from build123d import *

# Parameters (mm, degrees)
BOSS_EXTRUDE1_DEPTH      = 5
BOSS_EXTRUDE1_DEPTH_BACK = 2
SKETCH3_W                = 30
SKETCH3_H                = 10
BOSS_EXTRUDE2_DEPTH      = 25
SKETCH4_R                = 2.5
CUT_EXTRUDE1_DEPTH       = 83.331203834
RIB1_REACH               = 76.683
SKETCH6_WALL_W           = 186.72160491
SKETCH6_WALL_H           = 5
CUT_EXTRUDE2_DEPTH       = 7
CUT_EXTRUDE3_DEPTH       = 5
FILLET1_R                = 4
SKETCH9_R                = 1.75
CUT_EXTRUDE4_DEPTH       = 60.485369609
CHAMFER1_SIZE            = 1.6
FILLET2_R                = 4
SKETCH10_R               = 1.6
CUT_EXTRUDE5_DEPTH       = 52.293180378
CUT_EXTRUDE6_DEPTH       = 4
CHAMFER2_SIZE            = 1.6
FILLET3_R                = 2


with BuildPart() as part:
    # Sketch1 → Boss-Extrude1 (new, two sides)
    with BuildSketch(Plane.XY) as boss_extrude1_sk:
        Polygon((15, 27.5), (15, 12.5), (43.284271247, -15.784271247), (23.284271247, -35.784271247), (15, -27.5), (-15, -27.5), (-15, 27.5), align=None)
    extrude(amount=BOSS_EXTRUDE1_DEPTH)
    extrude(boss_extrude1_sk.sketch, amount=-BOSS_EXTRUDE1_DEPTH_BACK)

    # Sketch3 → Boss-Extrude2 (add)
    with BuildSketch(Plane.XY.offset(5)):
        with Locations((0, 22.5)):
            Rectangle(SKETCH3_W, SKETCH3_H)
    extrude(amount=BOSS_EXTRUDE2_DEPTH)

    # Sketch4 → Cut-Extrude1 (cut, through all)
    with BuildSketch(Plane(origin=(0, 27.5, 0), x_dir=(1, 0, 0), z_dir=(0, 1, 0))):
        with Locations(Location((-5, -13.9175, 0), (0, 0, 270))):
            Circle(SKETCH4_R)
    extrude(amount=-CUT_EXTRUDE1_DEPTH, mode=Mode.SUBTRACT)

    # Sketch6 wall → Rib1 (add, up to next)
    with BuildSketch(Plane(origin=(-15, 5, 17.5), x_dir=(0, -0.707106781187, -0.707106781187), z_dir=(0, -0.707106781187, 0.707106781187)), mode=Mode.PRIVATE) as rib1_sk1:
        with Locations((0, 2.5)):
            Rectangle(SKETCH6_WALL_W, SKETCH6_WALL_H)
    rib1_tool1 = extrude(rib1_sk1.sketch, amount=-RIB1_REACH, mode=Mode.PRIVATE) - part.part
    add(rib1_tool1.solids().sort_by_distance((-15, 5, 17.5))[0])

    # Sketch7 → Cut-Extrude2 (cut)
    with BuildSketch(Plane.XY.offset(5)):
        with BuildLine():
            Line((22.174744155, -18.158867896), (26.819805153, -32.248737342))
            Line((26.819805153, -32.248737342), (23.284271247, -35.784271247))
            Line((23.284271247, -35.784271247), (-15, -27.5))
            Line((-15, -27.5), (-15, -7.855339059))
            Line((-15, -7.855339059), (7.928932188, -7.855339059))
            ThreePointArc((7.928932188, -7.855339059), (16.719635588, -10.701182004), (22.174744155, -18.158867896))
        make_face()
    extrude(amount=-CUT_EXTRUDE2_DEPTH, mode=Mode.SUBTRACT)

    # Sketch8 → Cut-Extrude3 (cut)
    with BuildSketch(Plane(origin=(0, 17.5, 0), x_dir=(-1, 0, 0), z_dir=(0, -1, 0))):
        Polygon((0.265727793, -13.9175), (2.632863896, -18.0175), (7.367136104, -18.0175), (9.734272207, -13.9175), (7.367136104, -9.8175), (2.632863896, -9.8175), align=None)
    extrude(amount=-CUT_EXTRUDE3_DEPTH, mode=Mode.SUBTRACT)

    # Fillet1
    fillet1_edges = [part.edges().sort_by_distance(p)[0] for p in [
        (-15, 22.5, 30),
        (15, 22.5, 30),
    ]]
    fillet(fillet1_edges, radius=FILLET1_R)

    # Sketch9 → Cut-Extrude4 (cut, through all)
    with BuildSketch(Plane.XY.offset(5)):
        with Locations((15, -1.642135624)):
            Circle(SKETCH9_R)
        with Locations((29.142135624, -15.784271247)):
            Circle(SKETCH9_R)
        with Locations((-2.071067812, 2.5)):
            Circle(SKETCH9_R)
    extrude(amount=-CUT_EXTRUDE4_DEPTH, mode=Mode.SUBTRACT)

    # Chamfer1
    chamfer1_edges = [part.edges().sort_by_distance(p)[0] for p in [
        (-3.821067812, 2.5, 5),
        (27.392135624, -15.784271247, 5),
        (13.25, -1.642135624, 5),
    ]]
    chamfer(chamfer1_edges, length=CHAMFER1_SIZE)

    # Fillet2
    fillet2_edges = [part.edges().sort_by_distance(p)[0] for p in [
        (15, 12.5, 1.5),
        (43.284271247, -15.784271247, 1.5),
        (26.819805153, -32.248737342, 1.5),
        (-15, -7.855339059, 1.5),
    ]]
    fillet(fillet2_edges, radius=FILLET2_R)

    # Sketch10 → Cut-Extrude5 (cut, through all)
    with BuildSketch(Plane(origin=(15, 0, 0), x_dir=(0, 0, -1), z_dir=(1, 0, 0))):
        with Locations(Location((-7, 22.5, 0), (0, 0, 90))):
            Circle(SKETCH10_R)
    extrude(amount=-CUT_EXTRUDE5_DEPTH, mode=Mode.SUBTRACT)

    # Sketch11 → Cut-Extrude6 (cut)
    with BuildSketch(Plane.ZY.offset(15)):
        Polygon((8.58771324, 19.75), (10.175426481, 22.5), (8.58771324, 25.25), (5.41228676, 25.25), (3.824573519, 22.5), (5.41228676, 19.75), align=None)
    extrude(amount=-CUT_EXTRUDE6_DEPTH, mode=Mode.SUBTRACT)

    # Chamfer2
    chamfer2_edges = [part.edges().sort_by_distance(p)[0] for p in [
        (15, 20.9, 7),
    ]]
    chamfer(chamfer2_edges, length=CHAMFER2_SIZE)

    # Fillet3
    fillet3_edges = [part.edges().sort_by_distance(p)[0] for p in [
        (-10, 5, 5),
    ]]
    fillet(fillet3_edges, radius=FILLET3_R)


solid = part.part
Geometry check sheet. Reference: the model listing, model coordinates, mm. A direction names the side the tool comes from. Round coordinates to 2 decimals unless told otherwise and drop trailing zeros. Loops run counter-clockwise (first coordinate to the right, second up) from the corner with the lowest first, then second, coordinate; pieces in that order, holes last. Notation, with made-up numbers: (66.5, 46) - (111.5, 46) arc R20 ccw to (111.5, 74) - close; hole circle Ø5 at (54.5, 19). An arc over 180 degrees is marked (long way). One line per question, with ' | ' between items. Start each with the question number.
1. Depth check by flat-ended pin: pin 1 (12 mm diameter, centred on x = -3.5, z = 8.5, fed in from -Y); pin 2 (14 mm diameter, centred on x = 19.5, y = 3, fed in from +Z); pin 3 (10 mm diameter, centred on x = 3.5, z = 21, fed in from -Y); pin 4 (4 mm diameter, centred on x = -5, z = 13.92, fed in from +Y). Enter the tip coordinate at first touch or a pass-through.
2. Cross-section at D-D on z = 0.5. Record the cut outline in (x, y).
3. Cross-section at C-C on z = 23. Record the cut outline in (x, y), then the cut area to 3 significant figures.
4. Draft check along Z on faces 4 (the face through (-7, 22.5, 12)), 5 (the face through (0, 27.5, 14)), 6 (the face through (0, 23, 30)). Enter one of: released by +Z, released by -Z, zero draft, split by the parting line, or undercut.
5. Scan lines: line 1 (Z direction, x = 32, y = -9); line 2 (X direction, y = 15, z = 4); line 3 (X direction, y = 15, z = 9.5). Record each from-to range of solid material in increasing order. Write a range as [from, to].
6. Tool access check on faces 1 (the face through (-5, 20, 18.018)), 2 (the face through (-13, 19.75, 7)), 3 (the face through (-9.4, 4.82, 5.57)). Record the directions out of +Z, -Z, +X, -X, +Y, -Y that give a thin tool (end or side, any length) a straight path to the whole face; none if there is none.
7. Cross-section at B-B on z = 12.5. Record the cut outline in (x, y).
8. Cross-section at A-A on y = 2.5. Record the cut outline in (x, z).
Taken from the geometry:
1) pin 1: y = -7.86 | pin 2: z = 5 | pin 3: y = 17.5 | pin 4: through
2) outline: (-15, -3.86) arc R4 ccw to (-11, -7.86) - (7.93, -7.86) arc R15 cw to (22.17, -18.16) - (24.79, -26.08) arc R4 ccw to (31.41, -27.66) - (40.46, -18.61) arc R4 ccw to (40.46, -12.96) - (16.17, 11.33) arc R4 cw to (15, 14.16) - (15, 27.5) - (-15, 27.5) - close; hole circle Ø3.5 at (-2.07, 2.5); hole circle Ø3.5 at (15, -1.64); hole circle Ø3.5 at (29.14, -15.78)
3) outline: (-15, 10.5) - (-10, 10.5) - (-10, 17.5) - (15, 17.5) - (15, 27.5) - (-15, 27.5) - close | area: 335 mm²
4) face 4: undercut | face 5: zero draft | face 6: released by +Z
5) line 1: [-2, 5] | line 2: [-15, 15] | line 3: [-15, -10]
6) face 1: -Y | face 2: -X | face 3: +Z, +X, -Y
7) outline: (-15, 0) - (-10, 0) - (-10, 17.5) - (-8.92, 17.5) - (-8.92, 22.5) - (-7.06, 22.5) - (-7.06, 27.5) - (-15, 27.5) - close; (-2.94, 22.5) - (-1.08, 22.5) - (-1.08, 17.5) - (15, 17.5) - (15, 27.5) - (-2.94, 27.5) - close
8) outline: (-15, -2) - (-3.82, -2) - (-3.82, 3.4) - (-5.42, 5) - (-8, 5) arc R2 cw to (-10, 7) - (-10, 15) - (-15, 15) - close; (-0.32, -2) - (25, -2) - (25, 5) - (1.28, 5) - (-0.32, 3.4) - close
